Can you work these out from the model? Positions are in its coordinate system, mm. Face numbers are marked on the shaded views. Coordinates: 2 decimals unless noted, no trailing zeros. Loops run counter-clockwise (first coordinate to the right, second up) from the corner with the lowest first, then second, coordinate; pieces in that order, holes last. Notation, with made-up numbers: (51.5, 55.25) -> (89.5, 55.25) arc R35 ccw to (89.5, 94.25) -> close; hole circle Ø1 at (50.25, 40.5). An arc over 180 degrees is marked (long way). Use one line per item in the form item = value. Start each with the question number.
(1) Thinking about a two-plate mould opening in Y: for the marked faces 1, 2 and 3, which applies, released by +Y, released by -Y, zero draft, split by the parting line, or undercut?
(2) Imagine slicing it at C-C (y = 103). List the corners of the cut face in (x, z) for me, plus the area to 3 significant figures.
(3) I need wall thicknesses on line 1 (X direction, y = -149.5, z = -151); line 2 (Z direction, x = 1047.5, y = 177.5) (3 decimals); line 3 (Y direction, x = 662, z = -846.5). Which ranges of each line are inside material? Lowest first, please. Write a range as [from, to].
(4) Imagine slicing it at A-A (x = 972). List the corners of the cut face in (y, z) for me, plus the area to 3 significant figures.
(5) I'm going to push flat-ended pins straight in: pin 1 (6 mm diameter, centred on x = 856.5, z = -54, fed in from -Y); pin 2 (1 mm diameter, centred on x = 338, y = -365, fed in from +Z); pin 3 (10 mm diameter, centred on x = 984, z = -253, fed in from +Y). Where does each tip first touch, or does it pass through?
(6) Imagine slicing it at B-B (y = -635). State how many separate pieces and enclosed holes the cut face has, plus the area to 3 significant figures.
```python
from build123d import *

# Parameters (mm, degrees)
BOSS_EXTRUDE1_DEPTH = 1200
CUT_EXTRUDE1_DEPTH  = 1200
BOSS_EXTRUDE2_DEPTH = 20
BOSS_EXTRUDE6_DEPTH = 15


with BuildPart() as part:
    # Sketch1 → Boss-Extrude1 (new body)
    with BuildSketch(Plane(origin=(0, 0, 0), x_dir=(0, 0, -1), z_dir=(1, 0, 0))):
        Polygon((54.714181984, -127.878268169), (0, -100), (-196.261050551, 0), (-105.357341624, 178.408574129), (-183.765915753, 218.359738106), (-314.620788656, -38.457410151), (-39.951163977, -178.408574129), (54.714181984, -226.346681732), (1084.090701019, -750.840215293), (1123.92201101, -672.666867856), align=None)
    extrude(amount=BOSS_EXTRUDE1_DEPTH)

    # Sketch2 → Cut-Extrude1 (cut)
    with BuildSketch(Plane(origin=(0, -593.277605242, -1164.372860728), x_dir=(-1, 0, 0), z_dir=(0, -0.45399049973954697, -0.8910065241883679))):
        with BuildLine():
            ThreePointArc((-1076.711357012, -161.83665133), (-1035.853367703, -135.21654868), (-1020, -89.100652419))
            Line((-1020, -89.100652419), (-1170, -89.100652419))
            ThreePointArc((-1170, -89.100652419), (-1154.146632297, -135.21654868), (-1113.288642988, -161.83665133))
            Line((-1113.288642988, -161.83665133), (-1113.288642988, -176.83665133))
            Line((-1113.288642988, -176.83665133), (-1076.711357012, -176.83665133))
            Line((-1076.711357012, -176.83665133), (-1076.711357012, -161.83665133))
        make_face()
        with BuildLine():
            ThreePointArc((-911.711357012, -161.83665133), (-870.853367703, -135.21654868), (-855, -89.100652419))
            Line((-855, -89.100652419), (-1005, -89.100652419))
            ThreePointArc((-1005, -89.100652419), (-989.146632297, -135.21654868), (-948.288642988, -161.83665133))
            Line((-948.288642988, -161.83665133), (-948.288642988, -176.83665133))
            Line((-948.288642988, -176.83665133), (-911.711357012, -176.83665133))
            Line((-911.711357012, -176.83665133), (-911.711357012, -161.83665133))
        make_face()
        with BuildLine():
            ThreePointArc((-746.711357012, -161.83665133), (-705.853367703, -135.21654868), (-690, -89.100652419))
            Line((-690, -89.100652419), (-840, -89.100652419))
            ThreePointArc((-840, -89.100652419), (-824.146632297, -135.21654868), (-783.288642988, -161.83665133))
            Line((-783.288642988, -161.83665133), (-783.288642988, -176.83665133))
            Line((-783.288642988, -176.83665133), (-746.711357012, -176.83665133))
            Line((-746.711357012, -176.83665133), (-746.711357012, -161.83665133))
        make_face()
        with BuildLine():
            Line((-525, -89.100652419), (-675, -89.100652419))
            ThreePointArc((-675, -89.100652419), (-659.146632297, -135.21654868), (-618.288642988, -161.83665133))
            Line((-618.288642988, -161.83665133), (-618.288642988, -176.83665133))
            Line((-618.288642988, -176.83665133), (-581.711357012, -176.83665133))
            Line((-581.711357012, -176.83665133), (-581.711357012, -161.83665133))
            ThreePointArc((-581.711357012, -161.83665133), (-540.853367703, -135.21654868), (-525, -89.100652419))
        make_face()
        with BuildLine():
            Line((-360, -89.100652419), (-510, -89.100652419))
            ThreePointArc((-510, -89.100652419), (-494.146632297, -135.21654868), (-453.288642988, -161.83665133))
            Line((-453.288642988, -161.83665133), (-453.288642988, -176.83665133))
            Line((-453.288642988, -176.83665133), (-416.711357012, -176.83665133))
            Line((-416.711357012, -176.83665133), (-416.711357012, -161.83665133))
            ThreePointArc((-416.711357012, -161.83665133), (-375.853367703, -135.21654868), (-360, -89.100652419))
        make_face()
        with BuildLine():
            Line((-195, -89.100652419), (-345, -89.100652419))
            ThreePointArc((-345, -89.100652419), (-329.146632297, -135.21654868), (-288.288642988, -161.83665133))
            Line((-288.288642988, -161.83665133), (-288.288642988, -176.83665133))
            Line((-288.288642988, -176.83665133), (-251.711357012, -176.83665133))
            Line((-251.711357012, -176.83665133), (-251.711357012, -161.83665133))
            ThreePointArc((-251.711357012, -161.83665133), (-210.853367703, -135.21654868), (-195, -89.100652419))
        make_face()
        with BuildLine():
            Line((-30, -89.100652419), (-180, -89.100652419))
            ThreePointArc((-180, -89.100652419), (-164.146632297, -135.21654868), (-123.288642988, -161.83665133))
            Line((-123.288642988, -161.83665133), (-123.288642988, -176.83665133))
            Line((-123.288642988, -176.83665133), (-86.711357012, -176.83665133))
            Line((-86.711357012, -176.83665133), (-86.711357012, -161.83665133))
            ThreePointArc((-86.711357012, -161.83665133), (-45.853367703, -135.21654868), (-30, -89.100652419))
        make_face()
    extrude(amount=-CUT_EXTRUDE1_DEPTH, mode=Mode.SUBTRACT)

    # Sketch4 → Boss-Extrude2 (add)
    with BuildSketch(Plane.ZY):
        Polygon((196.261050551, 0), (128.16247559, 133.650978628), (-1192.020585971, -539.015889228), (-1123.92201101, -672.666867856), align=None)
    extrude(amount=-BOSS_EXTRUDE2_DEPTH)

    # Sketch14 → Boss-Extrude6 (add)
    with BuildSketch(Plane(origin=(1200, 0, 0), x_dir=(0, 0, -1), z_dir=(1, 0, 0))):
        Polygon((-196.261050551, 0), (-128.16247559, 133.650978628), (1192.020585971, -539.015889228), (1123.92201101, -672.666867856), align=None)
    extrude(amount=-BOSS_EXTRUDE6_DEPTH)


solid = part.part
```
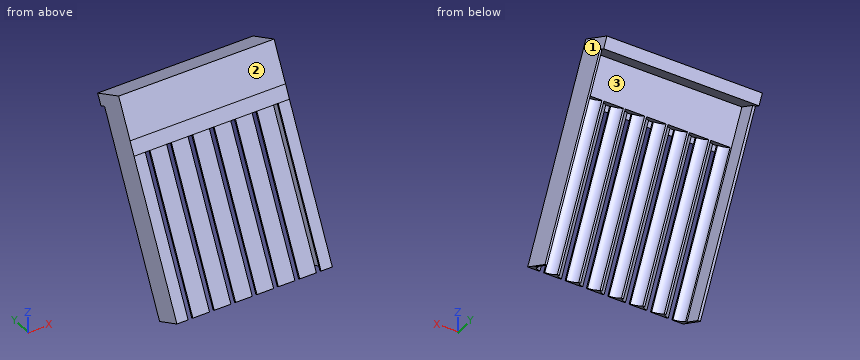
Worked out:
q1.face_1 = zero draft
q1.face_2 = released by -Y
q1.face_3 = undercut
q2.outline = (0, 68.01) -> (20, 68.01) -> (20, 143.78) -> (1185, 143.78) -> (1185, 68.01) -> (1200, 68.01) -> (1200, 242.54) -> (0, 242.54) -> close
q2.area = 121,000 mm2
q3.line_1 = [0, 20], [1185, 1200]
q3.line_2 = [105.82, 204.585]
q3.line_3 = [-629.78, -578.68]
q4.outline = (-750.84, -1084.09) -> (-728.03, -1095.71) -> (-183.24, -26.5) -> (-127.88, -54.71) -> (0, 196.26) -> (178.41, 105.36) -> (218.36, 183.77) -> (-38.46, 314.62) -> (-178.41, 39.95) -> (-226.35, -54.71) -> close
q4.area = 80,900 mm2
q5.pin_1 = -227.51
q5.pin_2 = -325.86
q5.pin_3 = -280.43
q6.separate_pieces = 8
q6.enclosed_holes = 0
q6.area = 91,300 mm2
